Work out the finished part from the listing and answer in its coordinate system (mm). A direction names the side the tool comes from. Round coordinates to 2 decimals unless told otherwise and drop trailing zeros. Order: outer loops, then holes, each group sorted by start corner. A loop starts at its lowest first (then second) coordinate and runs counter-clockwise, first axis right, second up. Notation, with made-up numbers: (-5.75, -17) - (24.25, -17) arc R17 cw to (24.25, -8) - close; hole circle Ø3 at (85, 75.25). An arc over 180 degrees is marked (long way). Use CSV: the item, a comma, the result in double quotes.
from build123d import *

# Parameters (mm, degrees)
SKICA1_W                 = 80
SKICA1_H                 = 25
P_IDAT_VYSUNUT_M1_DEPTH  = 25
SKICA2_W                 = 15
SKICA2_H                 = 5
ODEBRAT_VYSUNUT_M1_DEPTH = 51
ODEBRAT_VYSUNUT_M2_DEPTH = 8
ZKOSEN_1_SIZE            = 20
ZKOSEN_1_SIZE2           = 9.326153163
ODEBRAT_VYSUNUT_M3_DEPTH = 5
ODEBRAT_VYSUNUT_M4_DEPTH = 13
D_RA1_D                  = 5.5
D_RA1_DEPTH              = 25
D_RA1_CBORE_D            = 10
D_RA1_CBORE_DEPTH        = 5
D_RA1_TIP                = 1.652366702
M5_Z_VIT1_D              = 4.2
M5_Z_VIT1_DEPTH          = 14
M5_Z_VIT1_TIP            = 1.2618073
ZKOSEN_2_SIZE            = 1
ZAOBLIT1_R               = 0.5


with BuildPart() as part:
    # Skica1 → Přidat vysunutím1 (new body, symmetric)
    with BuildSketch(Plane.XY):
        Rectangle(SKICA1_W, SKICA1_H)
    extrude(amount=P_IDAT_VYSUNUT_M1_DEPTH, both=True)

    # Skica2 → Odebrat vysunutím1 (cut, through all)
    with BuildSketch(Plane.XY.offset(25)):
        with Locations((-32.5, -10)):
            Rectangle(SKICA2_W, SKICA2_H)
    extrude(amount=-ODEBRAT_VYSUNUT_M1_DEPTH, mode=Mode.SUBTRACT)

    # Skica3 → Odebrat vysunutím2 (cut)
    with BuildSketch(Plane(origin=(0, 12.5, 0), x_dir=(1, 0, 0), z_dir=(0, 1, 0))):
        Polygon((-40, 17.279404685), (-20, 10), (40, 10), (40, -10), (-20, -10), (-40, -17.279404685), align=None)
    extrude(amount=-ODEBRAT_VYSUNUT_M2_DEPTH, mode=Mode.SUBTRACT)

    # Zkosení1
    zkosen_1_edges = [part.edges().sort_by_distance(p)[0] for p in [
        (-40, 4.5, 0),
    ]]
    zkosen_1_side = [part.faces().sort_by_distance(p)[0] for p in [
        (-2.780115466, 4.5, 0),
    ]]
    chamfer(zkosen_1_edges, length=ZKOSEN_1_SIZE, length2=ZKOSEN_1_SIZE2, reference=zkosen_1_side[0])

    # Skica4 → Odebrat vysunutím3 (cut)
    with BuildSketch(Plane(origin=(0, 4.5, 0), x_dir=(1, 0, 0), z_dir=(0, 1, 0))):
        with BuildLine():
            Line((-3, 7), (23, 7))
            ThreePointArc((23, 7), (30, 0), (23, -7))
            Line((23, -7), (-3, -7))
            ThreePointArc((-3, -7), (-10, 0), (-3, 7))
        make_face()
    extrude(amount=-ODEBRAT_VYSUNUT_M3_DEPTH, mode=Mode.SUBTRACT)

    # Skica5 → Odebrat vysunutím4 (cut, through all)
    with BuildSketch(Plane(origin=(0, -0.5, 0), x_dir=(1, 0, 0), z_dir=(0, 1, 0))):
        with BuildLine():
            Line((-3, -4), (23, -4))
            ThreePointArc((23, -4), (27, 0), (23, 4))
            Line((23, 4), (-3, 4))
            ThreePointArc((-3, 4), (-7, 0), (-3, -4))
        make_face()
    extrude(amount=-ODEBRAT_VYSUNUT_M4_DEPTH, mode=Mode.SUBTRACT)

    # Díra1
    with Locations(Plane(origin=(0, 12.5, 0), x_dir=(1, 0, 0), z_dir=(0, 1, 0))):
        with Locations((-15, 17.5), (20, 17.5), (20, -17.5), (-15, -17.5)):
            CounterBoreHole(D_RA1_D / 2, D_RA1_CBORE_D / 2, D_RA1_CBORE_DEPTH, depth=D_RA1_DEPTH)
            with Locations((0, 0, -(D_RA1_DEPTH + D_RA1_TIP / 2))):  # 118° drill point
                Cone(0, D_RA1_D / 2, D_RA1_TIP, mode=Mode.SUBTRACT)

    # M5 závit1
    with Locations(Plane(origin=(40, 0, 0), x_dir=(0, 0, -1), z_dir=(1, 0, 0))):
        with Locations((-17.5, 5.5), (-17.5, -6.5), (17.5, 5.5), (17.5, -6.5)):
            Hole(M5_Z_VIT1_D / 2, depth=M5_Z_VIT1_DEPTH)
            with Locations((0, 0, -(M5_Z_VIT1_DEPTH + M5_Z_VIT1_TIP / 2))):  # 118° drill point
                Cone(0, M5_Z_VIT1_D / 2, M5_Z_VIT1_TIP, mode=Mode.SUBTRACT)

    # Zkosení2
    zkosen_2_edges = [part.edges().sort_by_distance(p)[0] for p in [
        (40, -6.5, -19.6),
        (40, 5.5, -19.6),
        (40, -6.5, 15.4),
        (40, 5.5, 15.4),
    ]]
    chamfer(zkosen_2_edges, length=ZKOSEN_2_SIZE)

    # Zaoblit1
    zaoblit1_edges = [part.edges().sort_by_distance(p)[0] for p in [
        (-10, -0.5, 0),
        (10, -0.5, -7),
        (30, -0.5, 0),
        (10, -0.5, 7),
    ]]
    fillet(zaoblit1_edges, radius=ZAOBLIT1_R)


solid = part.part
(1) Find section A-A (x = -15). Determine the outline of the cut face in (y, z).
Findings below:
outline,"(-12.5, -25) - (12.5, -25) - (12.5, -22.5) - (7.5, -22.5) - (7.5, -20.25) - (-12.5, -20.25) - close; (-12.5, -14.75) - (7.5, -14.75) - (7.5, -12.5) - (12.5, -12.5) - (12.5, -10) - (4.5, -10) - (4.5, 10) - (12.5, 10) - (12.5, 12.5) - (7.5, 12.5) - (7.5, 14.75) - (-12.5, 14.75) - close; (-12.5, 20.25) - (7.5, 20.25) - (7.5, 22.5) - (12.5, 22.5) - (12.5, 25) - (-12.5, 25) - close"
(2) Find section B-B (z = 0). Determine the outline of the cut face in (x, y), and give its area (3 significant figures).
Findings below:
outline,"(-40, -7.5) - (-25, -7.5) - (-25, -12.5) - (-7, -12.5) - (-7, -0.5) - (-9.5, -0.5) arc R0.5 cw to (-10, 0) - (-10, 4.5) - (-20, 4.5) - (-40, -4.83) - close; (27, -12.5) - (40, -12.5) - (40, 4.5) - (30, 4.5) - (30, 0) arc R0.5 cw to (29.5, -0.5) - (27, -0.5) - close"
area,"584 mm²"
(3) The mould has two halves that part along Y. Classify faces 5 (the cylindrical face through (32.409, -5.869, -15.497)), 6 (the flat face through (-1, 12.5, 18)), 7 (the flat face through (10, -6, -4)): released by +Y, released by -Y, zero draft, split by the parting line, or undercut.
Findings below:
face 5,"undercut"
face 6,"released by +Y"
face 7,"zero draft"
(4) Each of these flat-tipped pins is pushed along its axis until it touches: pin 1 (6 mm diameter, centred on x = 17.5, z = -2.5, fed in from +Y); pin 2 (4.5 mm diameter, centred on x = -32, z = 7.5, fed in from -Y); pin 3 (14.5 mm diameter, centred on x = 12, z = -2, fed in from +Y); pin 4 (3 mm diameter, centred on x = 19.5, z = -17, fed in from +Y). Where does it stop, or does it pass through?
Findings below:
pin 1,"stops at y = -0.5"
pin 2,"stops at y = -7.5"
pin 3,"stops at y = 4.5"
pin 4,"passes through"
(5) For faces 1 (the flat face through (-25, -10, 0)), 2 (the flat face through (10, 4.5, -9)), 3 (the cylindrical face through (-7, -6, 0)), 4 (the cylindrical face through (30, 2, 0)), determine the directions among +Z, -Z, +X, -X, +Y, -Y from which every point of the face is accessible in a straight line to the end or side of a thin tool.
Findings below:
face 1,"+Z, -Z, -X, -Y"
face 2,"+X, -X, +Y"
face 3,"+Y, -Y"
face 4,"+Y"
(6) Find section C-C (x = 10.5). Determine the outline of the cut face in (y, z).
Findings below:
outline,"(-12.5, -25) - (12.5, -25) - (12.5, -10) - (4.5, -10) - (4.5, -7) - (0, -7) arc R0.5 cw to (-0.5, -6.5) - (-0.5, -4) - (-12.5, -4) - close; (-12.5, 4) - (-0.5, 4) - (-0.5, 6.5) arc R0.5 cw to (0, 7) - (4.5, 7) - (4.5, 10) - (12.5, 10) - (12.5, 25) - (-12.5, 25) - close"
(7) Find section D-D (x = 20). State how many separate pieces and enclosed holes the cut face has, and give its area (3 significant figures).
Findings below:
separate pieces,"4"
enclosed holes,"0"
area,"604 mm²"
(8) Find the intervals of material crossed by L1, parallel to Z at x = 28.75, y = 5.5; L2, parallel to Z at x = 30.25, y = -6.5; L3, parallel to Z at x = 5.5, y = 1, in increasing order. Write a range as from..to.
Findings below:
L1,"z = -25..-19.6, -15.4..-10, 10..15.4, 19.6..25"
L2,"z = -25..-19.6, -15.4..15.4, 19.6..25"
L3,"z = -25..-7, 7..25"
